Input: part model. Units: mm. Frame: model coordinates. Face numbers are marked on the shaded views. Round coordinates to 2 decimals unless told otherwise and drop trailing zeros. Order: outer loops, then holes, each group sorted by start corner. A loop starts at its lowest first (then second) coordinate and runs counter-clockwise, first axis right, second up. Notation, with made-up numbers: (-24.5, -12.5) -> (10.5, -12.5) arc R10 ccw to (10.5, 6.5) -> close; hole circle Ø11 at (89.25, -3). An arc over 180 degrees is marked (long way). Use a Markdown table: item, result.
from build123d import *

# Parameters (mm, degrees)
SKETCH1_R           = 1.752344144
SKETCH1_R_2         = 3.25
BOSS_EXTRUDE1_DEPTH = 2
SCALE6_SCALE        = 2.8


with BuildPart() as part:
    # Sketch1 → Boss-Extrude1 (new body)
    with BuildSketch(Plane.XY):
        with BuildLine():
            Line((-201.779102887, 38.968850302), (-183.856871997, 38.968850302))
            ThreePointArc((-183.856871997, 38.968850302), (-179.50647719, 34.548425149), (-183.995805524, 30.26917))
            Line((-183.995805524, 30.26917), (-203.942326715, 30.587715102))
            Line((-203.942326715, 30.587715102), (-212.128411179, 30.587715102))
            ThreePointArc((-212.128411179, 30.587715102), (-216.977472251, 31.690715611), (-217.344366931, 36.650089735))
            Line((-217.344366931, 36.650089735), (-219.856871997, 48.906588317))
            Line((-219.856871997, 48.906588317), (-210.255760435, 42.440195681))
            Line((-210.255760435, 42.440195681), (-209.773273317, 43.15651595))
            Line((-209.773273317, 43.15651595), (-206.022177555, 40.564020545))
            add(Edge.make_bspline(
                [(-206.022177555, 40.564020545), (-204.845604067, 39.682708979), (-203.443834564, 39.1324171), (-201.779102887, 38.968850302)],
                knots=[0.24, 0.24, 0.24, 0.24, 0.28, 0.28, 0.28, 0.28], degree=3))
        make_face()
        with Locations((-183.856871997, 34.61790077)):
            Circle(SKETCH1_R, mode=Mode.SUBTRACT)
        with Locations((-213.807007526, 34.418525211)):
            Circle(SKETCH1_R_2, mode=Mode.SUBTRACT)
    extrude(amount=BOSS_EXTRUDE1_DEPTH)


with BuildPart() as part_1:
    # Scale6: scaled about (-200.816753652, 36.262830965, 1)
    add(part.part.scale(SCALE6_SCALE).moved(Location((361.470156574, -65.273095737, -1.8))))


solid = part_1.part
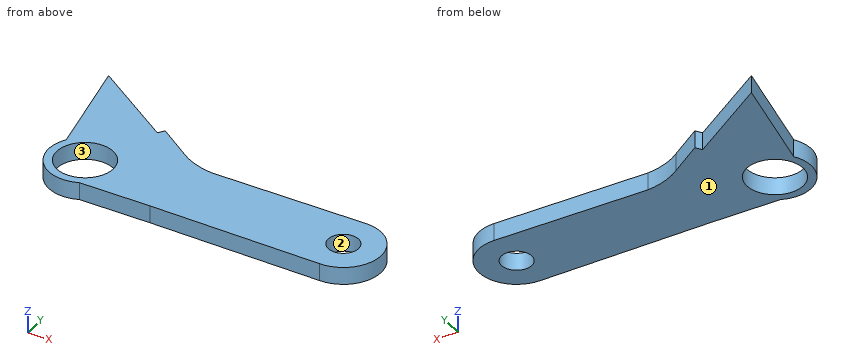
1) Cut plane C-C on y = 62. Return loops of the section in (x, z).
Answer key:
| item | result |
|---|---|
| outline | (-252.15, -1.8) -> (-239.78, -1.8) -> (-239.78, 3.8) -> (-252.15, 3.8) -> close |
2) Cut plane B-B on x = -181. Return loops of the section in (y, z).
Answer key:
| item | result |
|---|---|
| outline | (19.92, -1.8) -> (43.84, -1.8) -> (43.84, 3.8) -> (19.92, 3.8) -> close |
3) Ray query, probe 1 along X at (y, z) = (33, 3.1); probe 2 along X at (y, z) = (54, 1.4); probe 3 along Y at (x, z) = (-240.5, -0.6). Return the intervals inside material, ascending.
Answer key:
| item | result |
|---|---|
| probe 1 | x = -248.74 to -246.09, -228.29 to -158.05, -148.61 to -141.22 |
| probe 2 | x = -250.51 to -227.9, -226.95 to -223.63 |
| probe 3 | y = 19.87 to 22.62, 39.58 to 62.49 |
4) Contact query for flat-ended pins moving along their axis: P1, Ø3, axis at x = -189.5, z = 2, coming from the +Y side; P2, Ø21, axis at x = -237.19, y = 31.1, coming from the -Z side; P3, Ø2, axis at x = -219.5, z = 2, coming from the +Y side. Output: stop coordinate, or through.
Answer key:
| item | result |
|---|---|
| P1 | stops at y = 43.84 |
| P2 | stops at z = -1.8 |
| P3 | stops at y = 51.84 |
5) Cut plane D-D on z = 2. State how many separate pieces and enclosed holes the cut face has, and give its area (3 significant figures).
Answer key:
| item | result |
|---|---|
| separate pieces | 1 |
| enclosed holes | 2 |
| area | 2,680 mm^2 |
6) Cut plane A-A on y = 28. Return loops of the section in (x, z), and give its area (3 significant figures).
Answer key:
| item | result |
|---|---|
| outline | (-248.48, -1.8) -> (-245.75, -1.8) -> (-245.75, 3.8) -> (-248.48, 3.8) -> close; (-228.63, -1.8) -> (-156.6, -1.8) -> (-156.6, 3.8) -> (-228.63, 3.8) -> close; (-150.06, -1.8) -> (-141.71, -1.8) -> (-141.71, 3.8) -> (-150.06, 3.8) -> close |
| area | 465 mm^2 |
7) Draft query along X for the marked faces 1, 2 and 3. Return one class per face: released by +X, released by -X, zero draft, split by the parting line, or undercut.
Answer key:
| item | result |
|---|---|
| face 1 | zero draft |
| face 2 | undercut |
| face 3 | undercut |
